Print and shaded views of the part. All mm, measured from the part's lowest x, y and z. A direction names the side the tool comes from. Coordinates: 2 decimals unless noted, no trailing zeros. Loops run counter-clockwise (first coordinate to the right, second up) from the corner with the lowest first, then second, coordinate; pieces in that order, holes last.
1) Pin check, flat tips, straight feed: pin 1 Ø20 at (x, z) = (54, 38) entering from +Y; pin 2 Ø7 at (x, y) = (77, 8) entering from -Z; pin 3 Ø1.1 at (y, z) = (8.5, 0.5) entering from +X. Stop position of each tip, or through.
2) Saw through at B-B, the plane y = 12. Write the cut outline in (x, z), and give its area (3 significant figures).
3) Which spindle directions (+Z, -Z, +X, -X, +Y, -Y) get a long thin tool onto all of the face, cutting with end or side? Do the marked faces 4, 5 and 6. Say none if no direction does.
4) Saw through at A-A, the plane x = 30.5. Write the cut outline in (y, z).
5) Wall check: line 1 along X through (y, z) = (5.5, 27); line 2 along Z through (x, y) = (36.5, 2.25); line 3 along Z through (x, y) = (8.5, 4.25). Give the ranges that are in metal, low to high.
6) Two-plate mould, pull along X, no slides. Class the marked faces 1, 2 and 3: +X half, -X half, draft (parallel to the pull), parting line (faces both ways), or undercut.
7) Saw through at D-D, the plane x = 68.5. Write the cut outline in (y, z), and give its area (3 significant figures).
8) Saw through at C-C, the plane z = 28.5. Write the cut outline in (x, y), and give its area (3 significant figures).
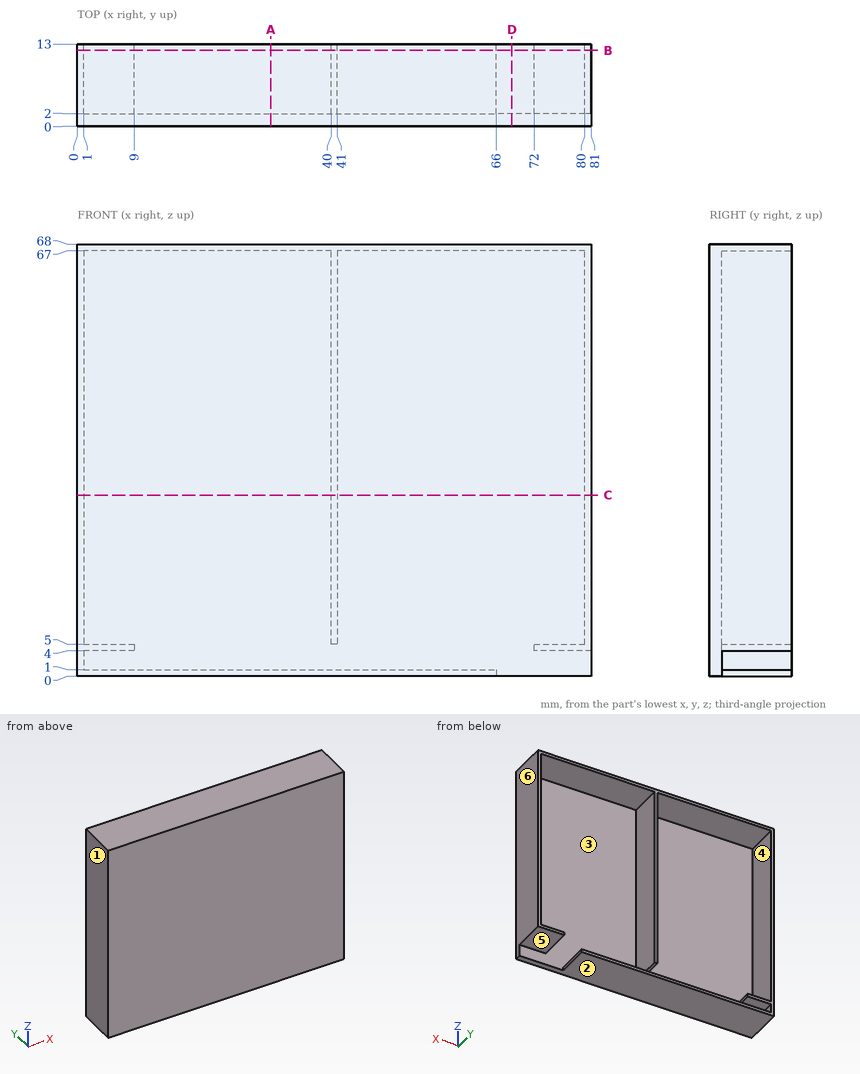
Data:
1. pin 1: stops at y = 2
1. pin 2: stops at z = 4
1. pin 3: stops at x = 66
2. outline: (0, 0) - (66, 0) - (66, 1) - (1, 1) - (1, 4) - (9, 4) - (9, 5) - (1, 5) - (1, 67) - (40, 67) - (40, 5) - (41, 5) - (41, 67) - (80, 67) - (80, 5) - (72, 5) - (72, 4) - (81, 4) - (81, 68) - (0, 68) - close
2. area: 354 mm2
3. face 4: +Y
3. face 5: -Z, +X, +Y
3. face 6: +Z, -Z, +X, +Y, -Y
4. outline: (0, 0) - (13, 0) - (13, 1) - (2, 1) - (2, 67) - (13, 67) - (13, 68) - (0, 68) - close
5. line 1: x = 0 to 1, 40 to 41, 80 to 81
5. line 2: z = 0 to 1, 67 to 68
5. line 3: z = 0 to 1, 4 to 5, 67 to 68
6. face 1: -X half
6. face 2: draft
6. face 3: undercut
7. outline: (0, 0) - (2, 0) - (2, 67) - (13, 67) - (13, 68) - (0, 68) - close
7. area: 147 mm2
8. outline: (0, 0) - (81, 0) - (81, 13) - (80, 13) - (80, 2) - (41, 2) - (41, 13) - (40, 13) - (40, 2) - (1, 2) - (1, 13) - (0, 13) - close
8. area: 195 mm2
